Here's how the part is built. I have some questions about the finished solid (model axes, mm). Face numbers are marked on the shaded views. A direction names the side the tool comes from. Coordinates: 2 decimals unless noted, no trailing zeros. Loops run counter-clockwise (first coordinate to the right, second up) from the corner with the lowest first, then second, coordinate; pieces in that order, holes last. Notation, with made-up numbers: M 56.25,63 L 72.25,63 A33 ccw 72.25,96 Z; hole C -16,8.5 d1. An arc over 180 degrees is marked long. Use one line per item in the form item = value. Start each with the question number.
(1) Please list where these lines run through material, in increasing order: L1, parallel to Z at x = -12.7, y = -2.1; L2, parallel to Y at x = -73.7, z = 25.4; L3, parallel to X at y = -1.45, z = 38.1.
(2) Imagine slicing it at C-C, the plane z = 12.7. Please give me the cut outline in (x, y) (3 decimals).
(3) Imagine slicing it at B-B, the plane x = -12.7. Please give me the cut outline in (y, z) (3 decimals).
(4) Will these pins go through, and if not, where does the flat tip stop? P1, Ø6.5, axis at y = -9, z = 31, coming from the +X side (3 decimals); P2, Ø3, axis at x = -12.7, z = 38.1, coming from the +Y side; P3, Ø4, axis at x = -69.92, z = 25.4, coming from the -Y side (3 decimals).
(5) On a 3-axis mill with a long thin cutter (end or side, diameter ignored), from which of +Z, -Z, +X, -X, +Y, -Y can I reach the whole of each face in a straight line? I mean the marked faces 1 and 2. Say none if no direction works.
(6) Imagine slicing it at D-D, the plane y = -15.24. Please give me the cut outline in (x, z) (3 decimals), and give its area (3 significant figures).
(7) Imagine slicing it at A-A, the plane z = 38.1. Please give me the cut outline in (x, y) (3 decimals), and give its area (3 significant figures).
```python
from build123d import *

# Parameters (mm, degrees)
BOSS_EXTRUDE1_DEPTH       = 76.2
TAP_DRILL_FOR_6_32_TAP1_D = 2.7051
TAP_DRILL_FOR_8_32_TAP1_D = 3.4544
CUT_EXTRUDE1_REACH        = 112.716
SKETCH8_W                 = 3.302
SKETCH8_H                 = 3.302
TAP_DRILL_FOR_8_32_TAP2_D = 3.4544


with BuildPart() as part:
    # Sketch2 → Boss-Extrude1 (new body)
    with BuildSketch(Plane.XY):
        Polygon((0, 0), (-76.2, 0), (-76.2, -25.4), (-73.025, -25.4), (-73.025, -3.175), (0, -3.175), align=None)
    extrude(amount=BOSS_EXTRUDE1_DEPTH)

    # Tap Drill for #6-32 Tap1 (through all)
    with Locations(Plane.ZY.offset(76.2)):
        with Locations((25.4, -15.24), (12.7, -15.24)):
            Hole(TAP_DRILL_FOR_6_32_TAP1_D / 2)

    # Tap Drill for #8-32 Tap1 (through all)
    with Locations(Plane(origin=(0, 0, 0), x_dir=(1, 0, 0), z_dir=(0, 1, 0))):
        with Locations((-69.917738612, -25.4), (-69.917738612, -50.8)):
            Hole(TAP_DRILL_FOR_8_32_TAP1_D / 2)

    # Sketch8 → Cut-Extrude1 (cut, up to next)
    with BuildSketch(Plane.ZY.offset(76.2), mode=Mode.PRIVATE) as cut_extrude1_sk1:
        with Locations((38.1, -15.24)):
            Rectangle(SKETCH8_W, SKETCH8_H)
    cut_extrude1_tool1 = extrude(cut_extrude1_sk1.sketch, amount=-CUT_EXTRUDE1_REACH, mode=Mode.PRIVATE) & part.part
    add(cut_extrude1_tool1.solids().sort_by_distance((-76.2, -15.24, 38.1))[0], mode=Mode.SUBTRACT)

    # Tap Drill for #8-32 Tap2 (through all)
    with Locations(Plane(origin=(0, 0, 0), x_dir=(1, 0, 0), z_dir=(0, 1, 0))):
        with Locations((-12.7, -19.05), (-12.7, -38.1), (-12.7, -57.15)):
            Hole(TAP_DRILL_FOR_8_32_TAP2_D / 2)


solid = part.part
```
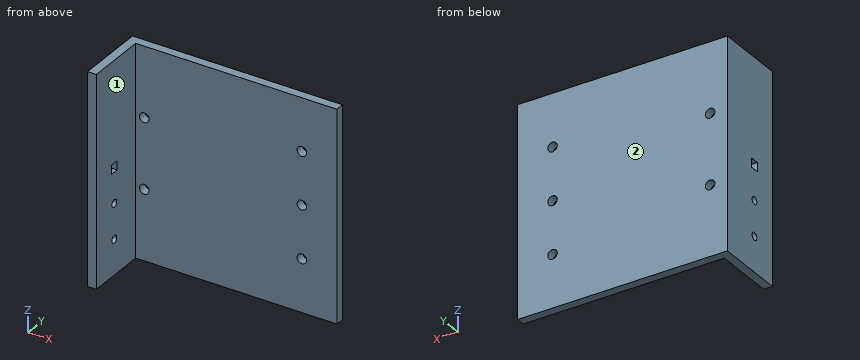
Answer:
q1.L1 = 0 to 17.32, 20.78 to 36.37, 39.83 to 55.42, 58.88 to 76.2
q1.L2 = -25.4 to -16.59, -13.89 to 0
q1.L3 = -76.2 to -14.43, -10.97 to 0
q2.outline = M -76.2,-25.4 L -73.025,-25.4 L -73.025,-16.593 L -76.2,-16.593 Z; M -76.2,-13.887 L -73.025,-13.887 L -73.025,-3.175 L 0,-3.175 L 0,0 L -76.2,0 Z
q3.outline = M -3.175,0 L 0,0 L 0,17.323 L -3.175,17.323 Z; M -3.175,20.777 L 0,20.777 L 0,36.373 L -3.175,36.373 Z; M -3.175,39.827 L 0,39.827 L 0,55.423 L -3.175,55.423 Z; M -3.175,58.877 L 0,58.877 L 0,76.2 L -3.175,76.2 Z
q4.P1 = -73.025
q4.P2 = through
q4.P3 = -3.175
q5.face_1 = +Z, -Z, +X, -Y
q5.face_2 = +Z, -Z, +X, -X, +Y
q6.outline = M -76.2,0 L -73.025,0 L -73.025,11.347 L -76.2,11.347 Z; M -76.2,14.053 L -73.025,14.053 L -73.025,24.047 L -76.2,24.047 Z; M -76.2,26.753 L -73.025,26.753 L -73.025,36.449 L -76.2,36.449 Z; M -76.2,39.751 L -73.025,39.751 L -73.025,76.2 L -76.2,76.2 Z
q6.area = 214 mm²
q7.outline = M -76.2,-25.4 L -73.025,-25.4 L -73.025,-16.891 L -76.2,-16.891 Z; M -76.2,-13.589 L -73.025,-13.589 L -73.025,-3.175 L -14.427,-3.175 L -14.427,0 L -76.2,0 Z; M -10.973,-3.175 L 0,-3.175 L 0,0 L -10.973,0 Z
q7.area = 291 mm²
